Here's how the part is built. I have some questions about the finished solid (model axes, mm). Face numbers are marked on the shaded views. A direction names the side the tool comes from. Round coordinates to 2 decimals unless told otherwise and drop trailing zeros. Order: outer loops, then holes, each group sorted by start corner. A loop starts at its lowest first (then second) coordinate and runs counter-clockwise, first axis right, second up.
```python
from build123d import *

# Parameters (mm, degrees)
SKETCH1_R           = 9.5
BOSS_EXTRUDE1_DEPTH = 11
SKETCH1_3_R         = 10.75
SKETCH1_3_R_2       = 9.5
BOSS_EXTRUDE2_DEPTH = 6.5
SKETCH3_R           = 1.75
CUT_EXTRUDE2_DEPTH  = 19.764994005
SKETCH4_R           = 1.75
CUT_EXTRUDE4_DEPTH  = 19.764994005
CUT_EXTRUDE5_START  = -8
SKETCH3_4_R         = 2.75
SKETCH3_4_R_2       = 1.75
CUT_EXTRUDE5_DEPTH  = 3


with BuildPart() as part:
    # Sketch1 → Boss-Extrude1 (new body)
    with BuildSketch(Plane.XY):
        Circle(SKETCH1_R)
    extrude(amount=-BOSS_EXTRUDE1_DEPTH)

    # Sketch1<3> → Boss-Extrude2 (add)
    with BuildSketch(Plane.XY):
        Circle(SKETCH1_3_R)
        Circle(SKETCH1_3_R_2, mode=Mode.SUBTRACT)
    extrude(amount=-BOSS_EXTRUDE2_DEPTH)

    # Sketch3 → Cut-Extrude2 (cut, through all)
    with BuildSketch(Plane(origin=(0, 0, -11), x_dir=(-1, 0, 0), z_dir=(0, 0, -1))):
        with Locations((0, 6.5)):
            Circle(SKETCH3_R)
        with Locations((-6.5, 0)):
            Circle(SKETCH3_R)
        with Locations((6.5, 0)):
            Circle(SKETCH3_R)
        with Locations((0, -6.5)):
            Circle(SKETCH3_R)
    extrude(amount=-CUT_EXTRUDE2_DEPTH, mode=Mode.SUBTRACT)

    # Sketch4 → Cut-Extrude4 (cut, through all)
    with BuildSketch(Plane(origin=(0, 0, -11), x_dir=(-1, 0, 0), z_dir=(0, 0, -1))):
        Circle(SKETCH4_R)
    extrude(amount=-CUT_EXTRUDE4_DEPTH, mode=Mode.SUBTRACT)

    # Sketch3<4> → Cut-Extrude5 (cut)
    # profile 1 of 4: a face of its own
    with BuildSketch(Plane(origin=(0, 0, -11), x_dir=(-1, 0, 0), z_dir=(0, 0, -1)).offset(CUT_EXTRUDE5_START)):
        with Locations(Location((-6.5, 0, 0), (0, 0, 180))):
            Circle(SKETCH3_4_R)
        with Locations((-6.5, 0)):
            Circle(SKETCH3_4_R_2, mode=Mode.SUBTRACT)
    # profile 2 of 4: a face of its own
    with BuildSketch(Plane(origin=(0, 0, -11), x_dir=(-1, 0, 0), z_dir=(0, 0, -1)).offset(CUT_EXTRUDE5_START)):
        with Locations(Location((0, 6.5, 0), (0, 0, 180))):
            Circle(SKETCH3_4_R)
        with Locations((0, 6.5)):
            Circle(SKETCH3_4_R_2, mode=Mode.SUBTRACT)
    # profile 3 of 4: a face of its own
    with BuildSketch(Plane(origin=(0, 0, -11), x_dir=(-1, 0, 0), z_dir=(0, 0, -1)).offset(CUT_EXTRUDE5_START)):
        with Locations(Location((6.5, 0, 0), (0, 0, 180))):
            Circle(SKETCH3_4_R)
        with Locations((6.5, 0)):
            Circle(SKETCH3_4_R_2, mode=Mode.SUBTRACT)
    # profile 4 of 4: a face of its own
    with BuildSketch(Plane(origin=(0, 0, -11), x_dir=(-1, 0, 0), z_dir=(0, 0, -1)).offset(CUT_EXTRUDE5_START)):
        with Locations(Location((0, -6.5, 0), (0, 0, 180))):
            Circle(SKETCH3_4_R)
        with Locations((0, -6.5)):
            Circle(SKETCH3_4_R_2, mode=Mode.SUBTRACT)
    extrude(amount=-CUT_EXTRUDE5_DEPTH, mode=Mode.SUBTRACT)


solid = part.part
```
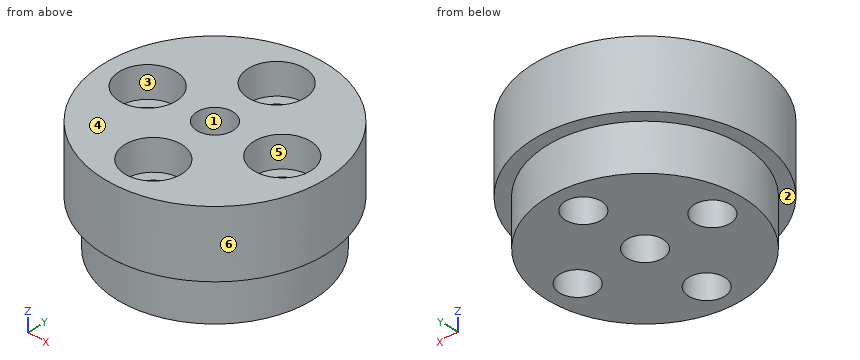
1. If we section it at B-B, the plane z = -2: Write out the boundary of the cut face in (x, y).
Evaluation:
outline: circle Ø21.5 at (0, 0); hole circle Ø5.5 at (-6.5, 0); hole circle Ø5.5 at (0, -6.5); hole circle Ø5.5 at (0, 6.5); hole circle Ø3.5 at (0, 0); hole circle Ø5.5 at (6.5, 0)
2. If we section it at A-A, the plane x = 0: Write out the boundary of the cut face in (y, z), and give its area (4 significant figures).
Evaluation:
outline: (-10.75, -6.5) - (-9.5, -6.5) - (-9.5, -11) - (-8.25, -11) - (-8.25, -3) - (-9.25, -3) - (-9.25, 0) - (-10.75, 0) - close; (-4.75, -11) - (-1.75, -11) - (-1.75, 0) - (-3.75, 0) - (-3.75, -3) - (-4.75, -3) - close; (1.75, -11) - (4.75, -11) - (4.75, -3) - (3.75, -3) - (3.75, 0) - (1.75, 0) - close; (8.25, -11) - (9.5, -11) - (9.5, -6.5) - (10.75, -6.5) - (10.75, 0) - (9.25, 0) - (9.25, -3) - (8.25, -3) - close
area: 97.75 mm2
3. If we section it at D-D, the plane x = -6.5: Write out the boundary of the cut face in (y, z), and give its area (3 significant figures).
Evaluation:
outline: (-8.56, -6.5) - (-6.93, -6.5) - (-6.93, -11) - (-1.75, -11) - (-1.75, -3) - (-2.75, -3) - (-2.75, 0) - (-8.56, 0) - close; (1.75, -11) - (6.93, -11) - (6.93, -6.5) - (8.56, -6.5) - (8.56, 0) - (2.75, 0) - (2.75, -3) - (1.75, -3) - close
area: 129 mm2
4. I'm going to push flat-ended pins straight in: P1, Ø3, axis at x = -6.5, y = 0, coming from the +Z side; P2, Ø4.5, axis at x = 0, y = 6.5, coming from the +Z side; P3, Ø5, axis at y = -8, z = -4.5, coming from the +X side; P4, Ø4, axis at x = -4, z = -7.5, coming from the -Y side. Where does each tip first touch, or does it pass through?
Evaluation:
P1: passes through
P2: stops at z = -3
P3: stops at x = 9.24
P4: stops at y = -10.51
5. On a 3-axis mill with a long thin cutter (end or side, diameter ignored), from which of +Z, -Z, +X, -X, +Y, -Y can I reach the whole of each face in a straight line? I mean the marked faces 1, 2 and 3. Say none if no direction works.
Evaluation:
face 1: +Z, -Z
face 2: -Z
face 3: +Z
6. If we mould it in two halves opening along Y, with no side actions, what happens to the marked faces 4, 5 and 6? For each: released by +Y, released by -Y, zero draft, split by the parting line, or undercut.
Evaluation:
face 4: zero draft
face 5: undercut
face 6: split by the parting line
7. I need wall thicknesses on probe 1 along Y at (x, z) = (0, -5); probe 2 along Y at (x, z) = (-0.5, -9); probe 3 along Z at (x, y) = (2.25, -5.25). Which ranges of each line are inside material? Lowest first, please.
Evaluation:
probe 1: y = -10.75 to -8.25, -4.75 to -1.75, 1.75 to 4.75, 8.25 to 10.75
probe 2: y = -9.49 to -8.18, -4.82 to -1.68, 1.68 to 4.82, 8.18 to 9.49
probe 3: z = -11 to -3
